Check sheet for the modelled part. Datum: model origin and axes. Units: mm. A direction names the side the tool comes from. Round coordinates to 2 decimals unless told otherwise and drop trailing zeros. Order: outer loops, then holes, each group sorted by start corner. A loop starts at its lowest first (then second) coordinate and runs counter-clockwise, first axis right, second up. Notation, with made-up numbers: (23.5, 65.25) -> (49.5, 65.25) arc R14 cw to (49.5, 88.25) -> close; hole circle Ø8 at (32.25, -32.5). An arc over 180 degrees is marked (long way). Use CSV: the item, a comma, the result in double quotes.
Autodesk Inventor part; units mm, degrees
ref_plane "YZ Plane" through (0, 0, 0) normal (1, 0, 0) x (0, 1, 0)
ref_plane "XZ Plane" through (0, 0, 0) normal (0, 1, 0) x (-1, 0, 0)
ref_plane "XY Plane" through (0, 0, 0) normal (0, 0, 1) x (1, 0, 0)
sketch "スケッチ1" plane through (0, 0, 0) normal (0, 1, 0) x (-1, 0, 0)
  line L0 (-10, 29) -> (10, 29)
  line L1 (10, 29) -> (10, -29)
  line L2 (10, -29) -> (-10, -29)
  line L3 (-10, -29) -> (-10, 29)
  point P0 (0, 0)
  dimension "d0" = 20
  dimension "d2" = 58
  dimension "d3" = 29
  dimension "d4" = 10
extrude "押し出し1" add sketch "スケッチ1" along normal blind 6
sketch "スケッチ2" plane through (-10, 0, 29) normal (0, 0, 1) x (1, 0, 0)
  line L0 (20, 0) -> (0, 0)
  line L1 (0, 0) -> (0, 6)
  circle A0 centre (5, 3) radius 1
  circle A1 centre (15, 3) radius 1
  point P0 (10, 0)
  dimension "d7" = 2
  dimension "d9" = 10
  dimension "d10" = 5
  dimension "d11" = 3
  dimension "d12" = 3
hole "穴1" at (5, 3, 29) at (-5, 3, 29) direction (0, 0, -1) diameter 1.6 depth 10 tip angle 118
sketch "スケッチ3" plane through (10, 0, -29) normal (0, 0, -1) x (-1, 0, 0)
  line L0 (20, 0) -> (0, 0)
  line L1 (0, 0) -> (0, 6)
  circle A0 centre (5, 3) radius 1
  circle A1 centre (15, 3) radius 1
  point P0 (10, 0)
  dimension "d20" = 2
  dimension "d22" = 3
  dimension "d23" = 3
  dimension "d24" = 10
  dimension "d25" = 5
hole "穴2" at (5, 3, -29) at (-5, 3, -29) direction (0, 0, 1) diameter 1.6 depth 10 tip angle 118
properties part number "Leg_Shim" material "アセタール樹脂、白"
Q1. Go/stop test with a flat-tipped pin: pin 1 (1.4 mm diameter, centred on x = -5, y = 3, fed in from -Z). Record where the tip stops, or that it passes through.
Result sheet:
pin 1,"stops at z = -18.94"
Q2. Sectioned sample at A-A, the plane z = 19.5. Enter the section's corners in (x, y), then the cut area to 3 significant figures.
Result sheet:
outline,"(-10, 0) -> (10, 0) -> (10, 6) -> (-10, 6) -> close; hole circle Ø1.6 at (-5, 3); hole circle Ø1.6 at (5, 3)"
area,"116 mm^2"
Q3. Mould release check, pull along X, two halves, no side actions. Record for faces 1 (the face through (4.92, 2.89, -18.6)), 2 (the face through (0, 0, 0)), 3 (the face through (-5.08, 3.11, 18.6)), 4 (the face through (10, 3, 0)): pulls with the +X half, pulls with the -X half, needs draft (parallel to the pull), parting line crosses it, or undercut.
Result sheet:
face 1,"undercut"
face 2,"needs draft"
face 3,"undercut"
face 4,"pulls with the +X half"
Q4. Scan lines: L1, parallel to X at y = 3, z = 22.5; L2, parallel to Y at x = -5, z = -21; L3, parallel to Y at x = 4.5, z = 23. Record each from-to range of solid material in increasing order.
Result sheet:
L1,"x = -10 to -5.8, -4.2 to 4.2, 5.8 to 10"
L2,"y = 0 to 2.2, 3.8 to 6"
L3,"y = 0 to 2.38, 3.62 to 6"
Q5. Access from +Z, -Z, +X, -X, +Y, -Y to the whole of each face (thin tool, end or side, straight path). Record for faces 5 (the face through (-4.29, 3.37, -23.93)), 6 (the face through (0, 3, -29)), 7 (the face through (-4.29, 2.63, 23.93)).
Result sheet:
face 5,"-Z"
face 6,"-Z, +X, -X, +Y, -Y"
face 7,"+Z"
